```python
from build123d import *

# Parameters (mm, degrees)
BOSS_EXTRUDE1_DEPTH          = 4
SKETCH3_R                    = 1.5
BOSS_EXTRUDE2_DEPTH          = 6
F_3_0_3_DIAMETER_HOLE1_D     = 3
F_3_0_3_DIAMETER_HOLE1_DEPTH = 10
F_4_0_4_DIAMETER_HOLE1_D     = 4
F_4_0_4_DIAMETER_HOLE1_DEPTH = 10
FILLET1_R                    = 2
FILLET2_R                    = 14.5
CUT_EXTRUDE1_DEPTH           = 73.945185819
CUT_EXTRUDE1_DEPTH_BACK      = 22
SKETCH8_R                    = 46
SKETCH9_R                    = 9.814954576
CUT_EXTRUDE2_DEPTH           = 21


with BuildPart() as part:
    # Sketch1 → Revolve1 (revolve)
    with BuildSketch(Plane(origin=(0, 0, 0), x_dir=(1, 0, 0), z_dir=(0, 1, 0))):
        Polygon((28, 45.5), (0, 45.5), (0, 16.5), (36, 16.5), (46, 26.5), (46, 40.5), align=None)
    revolve(axis=Axis((0, 0, -45.5), (0, 0, 1)))

    # Sketch2 → Boss-Extrude1 (add)
    with BuildSketch(Plane(origin=(0, 0, -45.5), x_dir=(-1, 0, 0), z_dir=(0, 0, -1))):
        Polygon((-9.814954576, 0), (-4.907477288, 8.5), (4.907477288, 8.5), (9.814954576, 0), (4.907477288, -8.5), (-4.907477288, -8.5), align=None)
    extrude(amount=BOSS_EXTRUDE1_DEPTH)

    # Sketch3 → Boss-Extrude2 (add)
    with BuildSketch(Plane.XY.offset(-16.5)):
        Circle(SKETCH3_R)
    extrude(amount=BOSS_EXTRUDE2_DEPTH)

    # Ø3.0 (3) Diameter Hole1
    with Locations(Plane.XY.offset(-16.5)):
        with Locations((-15.5, 0), (0, 15.5), (0, -15.5), (15.5, 0)):
            Hole(F_3_0_3_DIAMETER_HOLE1_D / 2, depth=F_3_0_3_DIAMETER_HOLE1_DEPTH)

    # Ø4.0 (4) Diameter Hole1
    with Locations(Plane(origin=(0, 0, -45.5), x_dir=(-1, 0, 0), z_dir=(0, 0, -1))):
        with Locations((0, -20), (-20, 0), (20, 0), (0, 20)):
            Hole(F_4_0_4_DIAMETER_HOLE1_D / 2, depth=F_4_0_4_DIAMETER_HOLE1_DEPTH)

    # Fillet1
    fillet1_edges = [part.edges().sort_by_distance(p)[0] for p in [
        (-46, 0, -40.5),
        (-46, 0, -26.5),
    ]]
    fillet(fillet1_edges, radius=FILLET1_R)

    # Fillet2
    fillet2_edges = [part.edges().sort_by_distance(p)[0] for p in [
        (-36, 0, -16.5),
    ]]
    fillet(fillet2_edges, radius=FILLET2_R)

    # Sketch8 → Cut-Extrude1 (cut, two sides: drawn at the far end of the back side and taken through both)
    with BuildSketch(Plane.XY.offset(-16.5).offset(-CUT_EXTRUDE1_DEPTH_BACK)):
        Circle(SKETCH8_R)
    extrude(amount=CUT_EXTRUDE1_DEPTH + CUT_EXTRUDE1_DEPTH_BACK, mode=Mode.SUBTRACT)

    # Sketch9 → Cut-Extrude2 (cut)
    with BuildSketch(Plane(origin=(0, 0, -49.5), x_dir=(-1, 0, 0), z_dir=(0, 0, -1))):
        Circle(SKETCH9_R)
    extrude(amount=-CUT_EXTRUDE2_DEPTH, mode=Mode.SUBTRACT)


solid = part.part
```
The model under review builds one solid part; all positions refer to its coordinate system, in mm. Round coordinates to 2 decimals unless told otherwise and drop trailing zeros. Loops run counter-clockwise (first coordinate to the right, second up) from the corner with the lowest first, then second, coordinate; pieces in that order, holes last. Notation, with made-up numbers: (20, -15.75) - (34, -15.75) arc R13 cw to (34, 8.25) - close; hole circle Ø1 at (44, -10.5). An arc over 180 degrees is marked (long way). Write each question's results on one line, items separated by ' | '. Start each with the question number.
Q1. Take a section at A-A on z = -42.25. Give the boundary of the cut face in (x, y).
Q2. Draft analysis for pull direction X (two halves, no side actions). For faces 1 (the cylindrical face through (7.234, 6.633, -42.049)), 2 (the flat face through (-1, 11, -38.5)), 3 (the conical face through (26.607, -11.032, -45.277)), 4 (the cylindrical face through (-21.6, -1.2, -42)), state which applies: pulls with the +X half, pulls with the -X half, needs draft (parallel to the pull), parting line crosses it, or undercut.
Q3. Insertion check: P1, Ø3, axis at x = 31.5, z = -41, coming from the +Y side; P2, Ø4, axis at x = -34, z = -42, coming from the -Y side; P3, Ø12, axis at x = -34, y = 2, coming from the -Z side. Each pin has a flat end and moves straight along its axis. Give the tip position at first contact, or say it passes through.
Q4. Wall thickness on line 1 along Y through (x, z) = (0, -40.5); line 2 along Y through (x, z) = (0, -40); line 3 along Z through (x, y) = (22, 27): over which ranges is each line inside the solid? List them lowest first. Write a range as [from, to].
Data:
1) outline: circle Ø79.4 at (0, 0); hole circle Ø4 at (-20, 0); hole circle Ø19.63 at (0, 0); hole circle Ø4 at (0, -20); hole circle Ø4 at (0, 20); hole circle Ø4 at (20, 0)
2) face 1: undercut | face 2: needs draft | face 3: parting line crosses it | face 4: undercut
3) P1: stops at y = 34.17 | P2: stops at y = -31.4 | P3: stops at z = -45.48
4) line 1: y = [-45.3, -22], [-18, -9.81], [9.81, 18], [22, 45.3] | line 2: y = [-45.72, -22], [-18, -9.81], [9.81, 18], [22, 45.72] | line 3: z = [-43.6, -38.5]
